from build123d import *

# Parameters (mm, degrees)
F0_W      = 35
F0_H      = 25
F0_R      = 1.75
F1_DEPTH  = 40
F2_W      = 35
F2_H      = 25
F3_DEPTH  = 23
F4_W      = 35
F4_H      = 5
F5_DEPTH  = 10
F6_W      = 35
F6_H      = 7
F7_DEPTH  = 10
F8_W      = 25
F8_H      = 7
F9_DEPTH  = 7
F10_W     = 14
F10_H     = 3
F11_DEPTH = 8
F15_DEPTH = 8
F16_W     = 21
F16_H     = 4
F17_DEPTH = 9
F18_DEPTH = 3


# Not quite as in the source:
# - a pattern or mirror of a feature is missing from the dataset's text; its kind, count and spacing are read off the source's solid


with BuildPart() as f1:
    # F0 (on Top) → F1 (new body)
    with BuildSketch(Plane.XY):
        Rectangle(F0_W, F0_H)
        with Locations((-12.5, -7.5)):
            Circle(F0_R, mode=Mode.SUBTRACT)
        with Locations((12.5, -7.5)):
            Circle(F0_R, mode=Mode.SUBTRACT)
        with Locations((-12.5, 7.5)):
            Circle(F0_R, mode=Mode.SUBTRACT)
        with Locations((12.5, 7.5)):
            Circle(F0_R, mode=Mode.SUBTRACT)
    extrude(amount=F1_DEPTH)

    # F2 (on face) → F3 (join)
    with BuildSketch(Plane.XY.offset(40)):
        Rectangle(F2_W, F2_H)
    extrude(amount=F3_DEPTH)

    # F4 (on face) → F5 (join)
    with BuildSketch(Plane.XY.offset(63)):
        with Locations((0, 10)):
            Rectangle(F4_W, F4_H)
    extrude(amount=F5_DEPTH)

    # F6 (on face) → F7 (join)
    with BuildSketch(Plane.XY.offset(63)):
        with Locations((0, -1)):
            Rectangle(F6_W, F6_H)
    extrude(amount=F7_DEPTH)

    # F8 (on face) → F9 (cut)
    with BuildSketch(Plane.XZ.offset(4.5)):
        with Locations((0, 66.5)):
            Rectangle(F8_W, F8_H)
    extrude(amount=-F9_DEPTH, mode=Mode.SUBTRACT)

    # F10 (on face) → F11 (join)
    with BuildSketch(Plane.XY.offset(63)):
        with Locations((0, -11)):
            Rectangle(F10_W, F10_H)
    extrude(amount=F11_DEPTH)

    # F14 (on offset) → F15 (cut)
    with BuildSketch(Plane.XY.offset(20)):
        Polygon((14.0011106999, -10.1), (15.5022213998, -7.5), (14.0011106999, -4.9), (10.9988893001, -4.9), (9.4977786002, -7.5), (10.9988893001, -10.1), align=None)
        Polygon((10.9988893001, 10.1), (9.4977786002, 7.5), (10.9988893001, 4.9), (14.0011106999, 4.9), (15.5022213998, 7.5), (14.0011106999, 10.1), align=None)
        Polygon((-10.9988893001, 4.9), (-9.4977786002, 7.5), (-10.9988893001, 10.1), (-14.0011106999, 10.1), (-15.5022213998, 7.5), (-14.0011106999, 4.9), align=None)
        Polygon((-14.0011106999, -10.1), (-10.9988893001, -10.1), (-9.4977786002, -7.5), (-10.9988893001, -4.9), (-14.0011106999, -4.9), (-15.5022213998, -7.5), align=None)
    extrude(amount=-F15_DEPTH, mode=Mode.SUBTRACT)

    # F16 (on face) → F17 (cut)
    with BuildSketch(Plane.YZ.offset(17.5)):
        with Locations((0, 18)):
            Rectangle(F16_W, F16_H)
    f17 = extrude(amount=-F17_DEPTH, mode=Mode.SUBTRACT)

    # F17_copies: F17 across plane
    add(f17.mirror(Plane(origin=(0, 0, 0), x_dir=(0, 0, -1), z_dir=(-1, 0, 0))), mode=Mode.SUBTRACT)

    # F12 (on face) → F18 (cut)
    with BuildSketch(Plane.XZ.offset(12.5)):
        Polygon((3.7173565517, 67), (1.8586782759, 70.2193252087), (-1.8586782759, 70.2193252087), (-3.7173565517, 67), (-1.8586782759, 63.7806747913), (1.8586782759, 63.7806747913), align=None)
    extrude(amount=-F18_DEPTH, mode=Mode.SUBTRACT)


solid = f1.part
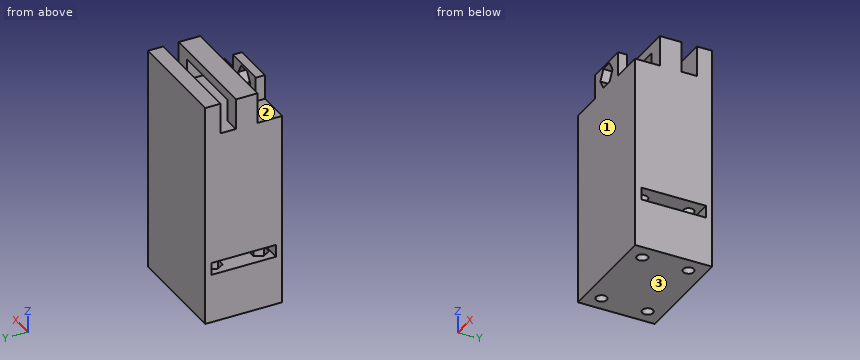
Here's how the part is built. I have some questions about the finished solid (model axes, mm). Face numbers are marked on the shaded views. Coordinates: 2 decimals unless noted, no trailing zeros. Order: outer loops, then holes, each group sorted by start corner. A loop starts at its lowest first (then second) coordinate and runs counter-clockwise, first axis right, second up. Notation, with made-up numbers: (41, -2) - (95, -2) arc R14 cw to (95, 18) - close; hole circle Ø4 at (72, 85.25). An arc over 180 degrees is marked (long way). Use CSV: the item, a comma, the result in double quotes. Start each with the question number.
1. If we mould it in two halves opening along Z, with no side actions, what happens to the marked faces 1, 2 and 3? For each: +Z half, -Z half, draft (parallel to the pull), parting line (faces both ways), or undercut.
2. Suppose I cut it at D-D on y = 3.5. List the corners of the cut face in (x, z) for me, then the cut area to 3 significant figures.
3. Suppose I cut it at B-B on z = 37.5. List the corners of the cut face in (x, y) for me, then the cut area to 3 significant figures.
4. Suppose I cut it at C-C on x = -3. List the corners of the cut face in (y, z) for me.
5. Suppose I cut it at A-A on y = -1.5. List the corners of the cut face in (x, z) for me, then the cut area to 3 significant figures.
6. Please list where these lines run through material, in increasing order: line 1 (Y direction, x = -12.5, z = 6.75); line 2 (X direction, y = 7.5, z = 32); line 3 (X direction, y = -6, z = 13). Write a range as from..to.
7. I'm going to push flat-ended pins straight in: pin 1 (3 mm diameter, centred on y = 3.5, z = 18, fed in from -X); pin 2 (1.5 mm diameter, centred on x = -3, y = -11.5, fed in from +Z); pin 3 (4.5 mm diameter, centred on x = -12.5, y = -7.5, fed in from +Z). Where does each tip first touch, or does it pass through?
Output:
1,face 1,"draft"
1,face 2,"undercut"
1,face 3,"-Z half"
2,outline,"(-17.5, 0) - (17.5, 0) - (17.5, 16) - (8.5, 16) - (8.5, 20) - (17.5, 20) - (17.5, 63) - (-17.5, 63) - (-17.5, 20) - (-8.5, 20) - (-8.5, 16) - (-17.5, 16) - close"
2,area,"2,130 mm2"
3,outline,"(-17.5, -12.5) - (17.5, -12.5) - (17.5, 12.5) - (-17.5, 12.5) - close; hole circle Ø3.5 at (-12.5, -7.5); hole circle Ø3.5 at (-12.5, 7.5); hole circle Ø3.5 at (12.5, -7.5); hole circle Ø3.5 at (12.5, 7.5)"
3,area,"837 mm2"
4,outline,"(-12.5, 0) - (12.5, 0) - (12.5, 73) - (7.5, 73) - (7.5, 63) - (-9.5, 63) - (-9.5, 65.76) - (-12.5, 65.76) - close; (-12.5, 68.24) - (-9.5, 68.24) - (-9.5, 71) - (-12.5, 71) - close; (-4.5, 70) - (2.5, 70) - (2.5, 73) - (-4.5, 73) - close"
5,outline,"(-17.5, 0) - (17.5, 0) - (17.5, 16) - (8.5, 16) - (8.5, 20) - (17.5, 20) - (17.5, 73) - (-17.5, 73) - (-17.5, 20) - (-8.5, 20) - (-8.5, 16) - (-17.5, 16) - close; hole (-12.5, 63) - (12.5, 63) - (12.5, 70) - (-12.5, 70) - close"
5,area,"2,310 mm2"
6,line 1,"y = -12.5..-9.25, -5.75..5.75, 9.25..12.5"
6,line 2,"x = -17.5..-14.25, -10.75..10.75, 14.25..17.5"
6,line 3,"x = -17.5..-14.64, -10.36..10.36, 14.64..17.5"
7,pin 1,"stops at x = -8.5"
7,pin 2,"stops at z = 71"
7,pin 3,"stops at z = 63"
